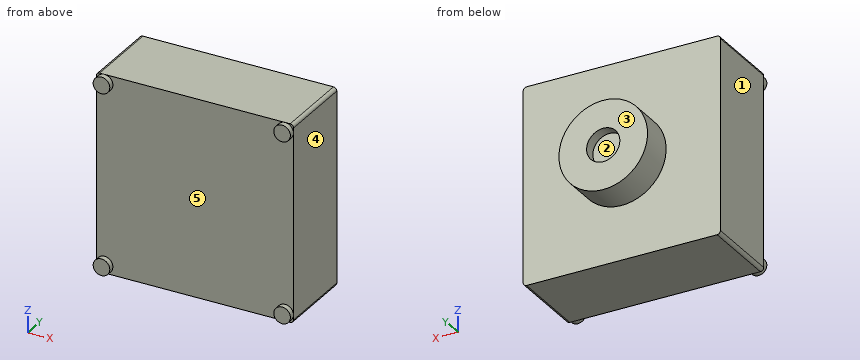
Autodesk Inventor part; units mm, degrees
ref_plane "YZ Plane" through (0, 0, 0) normal (1, 0, 0) x (0, 1, 0)
ref_plane "XZ Plane" through (0, 0, 0) normal (0, 1, 0) x (-1, 0, 0)
ref_plane "XY Plane" through (0, 0, 0) normal (0, 0, 1) x (1, 0, 0)
sketch "Sketch1" plane through (0, 0, 0) normal (0, 1, 0) x (-1, 0, 0)
  line L0 (89, -89) -> (-89, -89)
  line L1 (-89, -89) -> (-89, 89)
  line L2 (-89, 89) -> (89, 89)
  line L3 (89, 89) -> (89, -89)
  point P0 (0, 0)
  dimension "d0" = 89
  dimension "d1" = 178
  dimension "d2" = 178
  dimension "d3" = 89
extrude "Extrusion1" add sketch "Sketch1" along normal blind 70
sketch "Sketch2" plane through (0, 70, 0) normal (0, 1, 0) x (1, 0, 0)
  circle A0 centre (0, 0) radius 40
  dimension "d6" = 80
extrude "Extrusion2" add sketch "Sketch2" along normal blind 30
sketch "Sketch3" plane through (0, 100, 0) normal (0, 1, 0) x (1, 0, 0)
  circle A0 centre (0, 0) radius 15
  dimension "d9" = 30
extrude "Extrusion3" cut sketch "Sketch3" against normal blind 10
sketch "Sketch4" plane through (0, 0, 0) normal (0, -1, 0) x (1, 0, 0)
  circle A0 centre (-81.5, 81.5) radius 7.5
  line L0 (-89, 89) -> (89, 89)
  line L1 (-89, -89) -> (-89, 89)
  circle A1 centre (-81.5, -81.5) radius 7.5
  circle A2 centre (81.5, -81.5) radius 7.5
  circle A3 centre (81.5, 81.5) radius 7.5
  point P0 (0, 0)
  dimension "d12" = 15
  dimension "d13" = 7.5
  dimension "d14" = 7.5
  dimension "d17" = 360
extrude "Extrusion4" add sketch "Sketch4" along normal blind 5 contours A0 | A1 | A3 | A2
fillet "Fillet1" radius 3 4 edges at (-89, 35, 89) (89, 35, 89) (-89, 35, -89) (89, 35, -89)
properties part number "AERO - Base"
Source: CAD feature listing. Evaluate the final solid. Frame: model axes, mm. Face numbers are marked on the shaded views. A direction names the side the tool comes from. Give positions to 0.01 mm unless a question says otherwise; leave off trailing zeros. Write each loop counter-clockwise with the first axis right and the second up, starting at its lowest first coordinate (ties: lowest second). Pieces come first, ordered by that corner, then holes. Notation, with made-up numbers: (24, 34.25) -> (37, 34.25) arc R19 cw to (37, 61.25) -> close; hole circle Ø11 at (74.25, 23). An arc over 180 degrees is marked (long way). Return JSON: item names as keys, results as strings. Group by question number.
1. Section C-C, the plane y = 79.5. Output: boundary loops of the cut face in (x, z), then the cut area to 3 significant figures.
2. Access query for the marked faces 1 and 2. Directions: +Z, -Z, +X, -X, +Y, -Y. A direction counts if a zero-diameter tool reaches every point of the face in a straight line with its end or side. Return the directions, or none.
3. Section A-A, the plane x = 0. Output: boundary loops of the cut face in (y, z), then the cut area to 3 significant figures.
4. Pin query (flat end, axial travel): pin 1 Ø4 at (y, z) = (82, 15.5) entering from -X; pin 2 Ø5 at (x, z) = (53, -62) entering from -Y; pin 3 Ø4 at (y, z) = (87, 1) entering from -X. Return the tip coordinate at first contact, or that it passes through.
5. Material intervals for line 1 (Z direction, x = 0, y = 97); line 2 (Y direction, x = -74.5, z = -50.5), sorted ascending. Write a range as from..to.
6. Section B-B, the plane z = 0. Output: boundary loops of the cut face in (x, y), then the cut area to 3 significant figures.
7. Section D-D, the plane x = 32. Output: boundary loops of the cut face in (y, z).
8. Mould query, pull axis X, two halves, no side actions, for the marked faces 3, 4 and 5. Classes: +X half, -X half, draft (parallel to the pull), parting line (faces both ways), or undercut.
Determined:
{
 "1": {"outline": "circle Ø80 at (0, 0)", "area": "5,030 mm2"},
 "2": {"face 1": "+Z, -Z, -X, +Y, -Y", "face 2": "+Y"},
 "3": {"outline": "(0, -89) -> (70, -89) -> (70, -40) -> (100, -40) -> (100, -15) -> (90, -15) -> (90, 15) -> (100, 15) -> (100, 40) -> (70, 40) -> (70, 89) -> (0, 89) -> close", "area": "14,600 mm2"},
 "4": {"pin 1": "stops at x = -37.65", "pin 2": "stops at y = 0", "pin 3": "stops at x = -40"},
 "5": {"line 1": "z = -40..-15, 15..40", "line 2": "y = 0..70"},
 "6": {"outline": "(-89, 0) -> (89, 0) -> (89, 70) -> (40, 70) -> (40, 100) -> (15, 100) -> (15, 90) -> (-15, 90) -> (-15, 100) -> (-40, 100) -> (-40, 70) -> (-89, 70) -> close", "area": "14,600 mm2"},
 "7": {"outline": "(0, -89) -> (70, -89) -> (70, -24) -> (100, -24) -> (100, 24) -> (70, 24) -> (70, 89) -> (0, 89) -> close"},
 "8": {"face 3": "draft", "face 4": "+X half", "face 5": "undercut"}
}
